Part print with two shaded views. Sizes in mm from the minimum x, y, z corner. A direction names the side the tool comes from. Coordinates: 2 decimals unless noted, no trailing zeros. Write each loop counter-clockwise with the first axis right and the second up, starting at its lowest first coordinate (ties: lowest second). Pieces come first, ordered by that corner, then holes.
Q1. Band-saw the part on A-A, the plane y = 21. Write the cut outline in (x, z).
Q2. Band-saw the part on D-D, the plane z = 39. Write the cut outline in (x, y).
Q3. Band-saw the part on C-C, the plane z = 28.5. Write the cut outline in (x, y), plus the area to 3 significant figures.
Q4. Pin check, flat tips, straight feed: P1, Ø8, axis at y = 19.5, z = 26, coming from the +X side; P2, Ø10, axis at x = 33.5, y = 28, coming from the +Z side; P3, Ø5, axis at y = 27, z = 12.5, coming from the +X side; P4, Ø1.5, axis at x = 29.5, z = 45.5, coming from the +Y side. Stop position of each tip, or through.
Q5. Which spindle directions (+Z, -Z, +X, -X, +Y, -Y) get a long thin tool onto all of the face, cutting with end or side? Do the marked faces 1 and 2. Say none if no direction does.
Q6. Drill centre lines: probe 1 along Z at (x, y) = (39, 18); probe 2 along Z at (x, y) = (33, 20); probe 3 along X at (y, z) = (10, 21). Where is each one in solid material? Low to high.
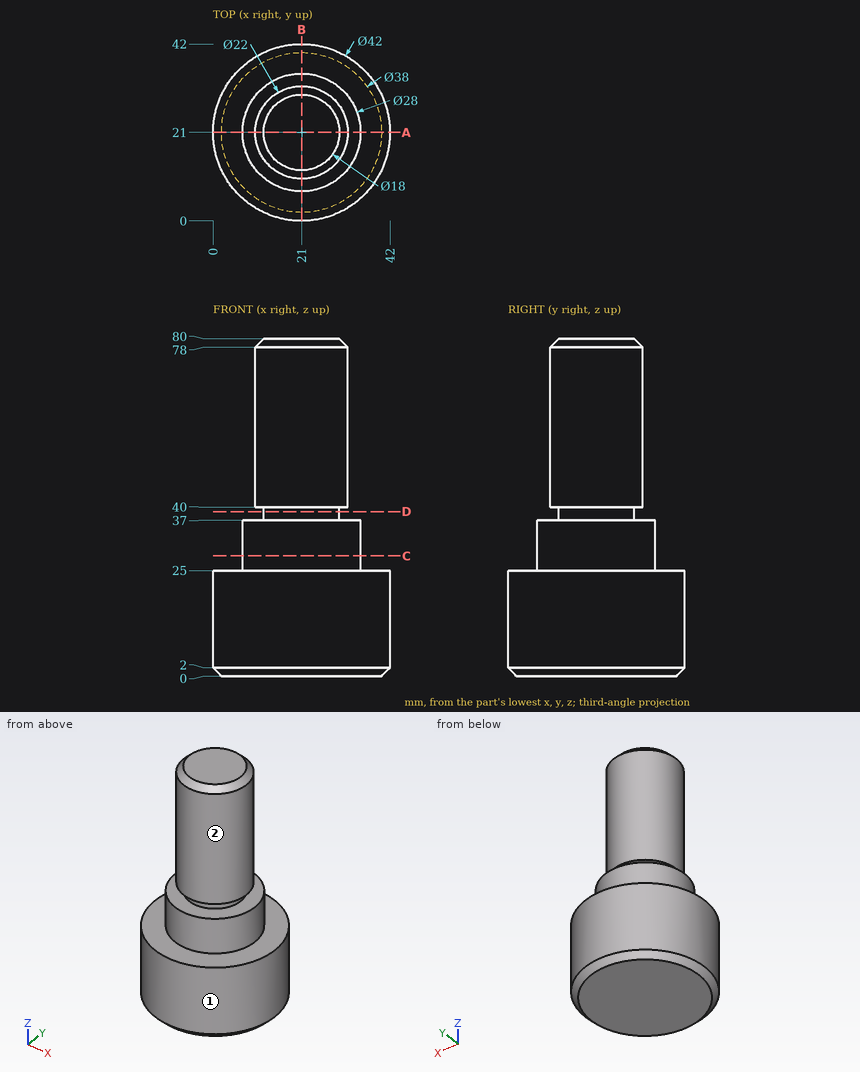
Answer sheet:
1. outline: (0, 2) - (2, 0) - (40, 0) - (42, 2) - (42, 25) - (35, 25) - (35, 37) - (30, 37) - (30, 40) - (32, 40) - (32, 78) - (30, 80) - (12, 80) - (10, 78) - (10, 40) - (12, 40) - (12, 37) - (7, 37) - (7, 25) - (0, 25) - close
2. outline: circle Ø18 at (21, 21)
3. outline: circle Ø28 at (21, 21)
3. area: 616 mm2
4. P1: stops at x = 42
4. P2: stops at z = 79.67
4. P3: stops at x = 41.71
4. P4: stops at y = 28.81
5. face 1: +Z, -Z
5. face 2: +Z
6. probe 1: z = 0 to 25
6. probe 2: z = 0 to 37
6. probe 3: x = 3.11 to 38.89
